Autodesk Inventor part; units mm, degrees
ref_plane "YZ Plane" through (0, 0, 0) normal (1, 0, 0) x (0, 1, 0)
ref_plane "XZ Plane" through (0, 0, 0) normal (0, 1, 0) x (-1, 0, 0)
ref_plane "XY Plane" through (0, 0, 0) normal (0, 0, 1) x (1, 0, 0)
sketch "Sketch1" plane through (0, 0, 0) normal (0, 0, 1) x (1, 0, 0)
  line L0 (-29.75, -11.25) -> (29.75, -11.25)
  line L1 (29.75, -11.25) -> (29.75, 11.25)
  line L2 (29.75, 11.25) -> (-29.75, 11.25)
  line L3 (-29.75, 11.25) -> (-29.75, -11.25)
  line L4 (-29.75, -11.25) -> (29.75, 11.25) construction
  line L5 (29.75, -11.25) -> (-29.75, 11.25) construction
  point P0 (0, 0)
  dimension "d0" = 59.5
  dimension "d1" = 22.5
extrude "Extrusion1" add sketch "Sketch1" against normal blind 1.6
fillet "Fillet1" radius 1 4 edges at (29.75, 11.25, -0.8) (-29.75, 11.25, -0.8) (29.75, -11.25, -0.8) (-29.75, -11.25, -0.8)
sketch "Sketch2" plane through (0, 0, 0) normal (0, 0, 1) x (1, 0, 0)
  line L0 (-21.9, 4.1) -> (-20.1, 4.1)
  line L1 (-20.1, 4.1) -> (-20.1, 0.9)
  line L2 (-20.1, 0.9) -> (-21.9, 0.9)
  line L3 (-21.9, 0.9) -> (-21.9, 4.1)
  line L4 (-21.9, 4.1) -> (-20.1, 0.9) construction
  line L5 (-20.1, 4.1) -> (-21.9, 0.9) construction
  line L6 (-20.1, -0.9) -> (-21.9, -0.9)
  line L7 (-21.9, -0.9) -> (-21.9, -4.1)
  line L8 (-21.9, -4.1) -> (-20.1, -4.1)
  line L9 (-20.1, -4.1) -> (-20.1, -0.9)
  line L10 (-20.1, -0.9) -> (-21.9, -4.1) construction
  line L11 (-21.9, -0.9) -> (-20.1, -4.1) construction
  line L12 (-17, 0) -> (-17, 5.3945) construction
  line L13 (-12.1, 4.1) -> (-13.9, 4.1)
  line L14 (-13.9, 4.1) -> (-13.9, 0.9)
  line L15 (-13.9, 0.9) -> (-12.1, 0.9)
  line L16 (-12.1, 0.9) -> (-12.1, 4.1)
  line L17 (-12.1, 4.1) -> (-13.9, 0.9) construction
  line L18 (-13.9, 4.1) -> (-12.1, 0.9) construction
  line L19 (-13.9, -0.9) -> (-12.1, -0.9)
  line L20 (-12.1, -0.9) -> (-12.1, -4.1)
  line L21 (-12.1, -4.1) -> (-13.9, -4.1)
  line L22 (-13.9, -4.1) -> (-13.9, -0.9)
  line L23 (-13.9, -0.9) -> (-12.1, -4.1) construction
  line L24 (-12.1, -0.9) -> (-13.9, -4.1) construction
  line L25 (-29.75, 10.25) -> (-29.75, -10.25)
  line L26 (-28.75, -11.25) -> (28.75, -11.25)
  point P0 (0, 0)
  point P1 (-21, 2.5)
  point P2 (-21, -2.5)
  point P3 (-13, 2.5)
  point P4 (-13, -2.5)
  dimension "d5" = 17
  dimension "d6" = 1.8
  dimension "d7" = 0.9
  dimension "d8" = 0
  dimension "d10" = 1.8
  dimension "d11" = 1.8
  dimension "d12" = 3.2
  dimension "d13" = 3.2
  dimension "d16" = 4
  dimension "d17" = 8.75
  dimension "d28" = 11.25
  dimension "d29" = 16.75
extrude "Extrusion2" cut sketch "Sketch2" against normal blind 1.6
sketch "Sketch3" plane through (0, 0, 0) normal (0, 0, 1) x (1, 0, 0)
  line L0 (-29.75, 10.25) -> (-29.75, -10.25) construction
  line L1 (16, 5) -> (16, -5) construction
  circle A0 centre (16, 5) radius 3.5
  circle A1 centre (16, -5) radius 3
  line L2 (-28.75, -11.25) -> (28.75, -11.25)
  point P0 (0, 0)
  dimension "d18" = 7
  dimension "d19" = 6
  dimension "d20" = 10
  dimension "d21" = 5
  dimension "d22" = 16
  dimension "d25" = 45.75
  dimension "d26" = 6.25
  dimension "d27" = 16.25
extrude "Extrusion3" cut sketch "Sketch3" against normal through all
sketch "Sketch4" plane through (0, 0, 0) normal (0, 0, 1) x (1, 0, 0)
  line L0 (-29.75, 11.25) -> (29.75, 11.25) construction
  line L1 (29.75, 11.25) -> (29.75, -11.2319) construction
  line L2 (29.75, -11.2319) -> (-29.75, -11.2319) construction
  line L3 (-29.75, -11.2319) -> (-29.75, 11.25) construction
  line L4 (28.75, 11.25) -> (-28.75, 11.25)
  line L5 (-29.75, 10.25) -> (-29.75, -10.25)
  line L6 (29.75, -10.25) -> (29.75, 10.25)
  point P0 (0, 0)
decal "Decal1"
sketch "Sketch5" plane through (0, 0, -1.6) normal (0, 0, -1) x (-1, 0, 0)
  line L0 (-29.75, 11.25) -> (29.75, 11.25) construction
  line L1 (29.75, 11.25) -> (29.75, -11.2319) construction
  line L2 (29.75, -11.2319) -> (-29.75, -11.2319) construction
  line L3 (-29.75, -11.2319) -> (-29.75, 11.25) construction
  line L4 (28.75, 11.25) -> (-28.75, 11.25)
  line L5 (-29.75, 10.25) -> (-29.75, -10.25)
  line L6 (29.75, -10.25) -> (29.75, 10.25)
  point P0 (0, 0)
decal "Decal2"
equation "\"d7\" = 0.5 * d6"
properties part number "KeyerFront_Iambic"
Can you work these out from the model? Positions are in its coordinate system, mm. A direction names the side the tool comes from. Coordinates: 2 decimals unless noted, no trailing zeros. Order: outer loops, then holes, each group sorted by start corner. A loop starts at its lowest first (then second) coordinate and runs counter-clockwise, first axis right, second up. Notation, with made-up numbers: M 36.5,58.5 L 54.5,58.5 A17 cw 54.5,87.5 Z; hole C 0,29.25 d10. An arc over 180 degrees is marked long. Answer as CSV lines item,"result".
(1) Suppose I cut it at C-C on z = -0.85. Please give me the cut outline in (x, y), plus the area to 3 significant figures.
Geometry check:
outline,"M -29.75,-10.25 A1 ccw -28.75,-11.25 L 28.75,-11.25 A1 ccw 29.75,-10.25 L 29.75,10.25 A1 ccw 28.75,11.25 L -28.75,11.25 A1 ccw -29.75,10.25 Z; hole M -21.9,-4.1 L -20.1,-4.1 L -20.1,-0.9 L -21.9,-0.9 Z; hole M -21.9,0.9 L -20.1,0.9 L -20.1,4.1 L -21.9,4.1 Z; hole M -13.9,-4.1 L -12.1,-4.1 L -12.1,-0.9 L -13.9,-0.9 Z; hole M -13.9,0.9 L -12.1,0.9 L -12.1,4.1 L -13.9,4.1 Z; hole C 16,5 d7; hole C 16,-5 d6"
area,"1,250 mm^2"
(2) Please list where these lines run through material, in increasing order: L1, parallel to Y at x = 16, z = -0.95; L2, parallel to X at y = -2.25, z = -0.4; L3, parallel to X at y = 4.75, z = -1.3.
Geometry check:
L1,"-11.25 to -8, -2 to 1.5, 8.5 to 11.25"
L2,"-29.75 to -21.9, -20.1 to -13.9, -12.1 to 14.8, 17.2 to 29.75"
L3,"-29.75 to 12.51, 19.49 to 29.75"
(3) Suppose I cut it at A-A on x = 16. Please give me the cut outline in (y, z).
Geometry check:
outline,"M -11.25,-1.6 L -8,-1.6 L -8,0 L -11.25,0 Z; M -2,-1.6 L 1.5,-1.6 L 1.5,0 L -2,0 Z; M 8.5,-1.6 L 11.25,-1.6 L 11.25,0 L 8.5,0 Z"
(4) Suppose I cut it at B-B on y = -5. Please give me the cut outline in (x, z).
Geometry check:
outline,"M -29.75,-1.6 L 13,-1.6 L 13,0 L -29.75,0 Z; M 19,-1.6 L 29.75,-1.6 L 29.75,0 L 19,0 Z"
(5) On a 3-axis mill with a long thin cutter (end or side, diameter ignored), from which of +Z, -Z, +X, -X, +Y, -Y can I reach the whole of each face in a straight line? I mean faces 4 (the flat face through (-12.1, -2, -1)), 5 (the cylindrical face through (-29.449, -10.965, -0.811)). Say none if no direction works.
Geometry check:
face 4,"+Z, -Z"
face 5,"+Z, -Z, -X, -Y"
(6) I'm going to push a flat-ended pin straight in: pin 1 (8 mm diameter, centred on x = -21, y = -1, fed in from -Z). Where does the tip first touch, or does it pass through?
Geometry check:
pin 1,"z = -1.6"
(7) Suppose I cut it at D-D on y = 5. Please give me the cut outline in (x, z), plus the area to 3 significant figures.
Geometry check:
outline,"M -29.75,-1.6 L 12.5,-1.6 L 12.5,0 L -29.75,0 Z; M 19.5,-1.6 L 29.75,-1.6 L 29.75,0 L 19.5,0 Z"
area,"84.0 mm^2"
(8) If we mould it in two halves opening along Y, with no side actions, what happens to faces 1 (the flat face through (0, 0, 0)), 2 (the cylindrical face through (29.465, -10.949, -0.811)), 3 (the flat face through (-13, 4.1, -1))? For each: released by +Y, released by -Y, zero draft, split by the parting line, or undercut.
Geometry check:
face 1,"zero draft"
face 2,"released by -Y"
face 3,"undercut"
